The model under review builds one solid part; all positions refer to its coordinate system, in mm. Coordinates: 2 decimals unless noted, no trailing zeros. Order: outer loops, then holes, each group sorted by start corner. A loop starts at its lowest first (then second) coordinate and runs counter-clockwise, first axis right, second up. Notation, with made-up numbers: (74.25, 89.25) - (125.25, 89.25) arc R21 ccw to (125.25, 94.25) - close; hole circle Ø5 at (-26.5, 66). An arc over 180 degrees is marked (long way). Answer in a Markdown table with one row per item.
Autodesk Inventor part; units mm, degrees
ref_plane "YZ Plane" through (0, 0, 0) normal (1, 0, 0) x (0, 1, 0)
ref_plane "XZ Plane" through (0, 0, 0) normal (0, 1, 0) x (-1, 0, 0)
ref_plane "XY Plane" through (0, 0, 0) normal (0, 0, 1) x (1, 0, 0)
sketch "Sketch1" plane through (0, 0, 0) normal (0, 0, 1) x (1, 0, 0)
  line L0 (0, 3.85) -> (0, -3.85)
  line L1 (0, -3.85) -> (4, -3.85)
  line L2 (4, -3.85) -> (4, 3.85)
  line L3 (4, 3.85) -> (0, 3.85)
  arc A0 (0, -5.5518) -> (0, 5.5518) centre (0, 0) ccw
  line L4 (0, 5.5518) -> (0, -5.5518)
  line L5 (4, 5.5518) -> (6, 5.5518)
  line L6 (6, 5.5518) -> (6, -5.5518)
  line L7 (6, -5.5518) -> (4, -5.5518)
  line L8 (4, -5.5518) -> (4, 5.5518)
  line L9 (0, 2.5) -> (6, 2.5)
  line L10 (6, 2.5) -> (6, 0)
  line L11 (6, 0) -> (0, 0)
  line L12 (0, 0) -> (0, 2.5)
  dimension "d0" = 7.7
  dimension "d2" = 4
  dimension "d3" = 3.85
  dimension "d4" = 2
  dimension "d5" = 2
  dimension "d6" = 6
  dimension "d7" = 6
  dimension "d8" = 2.5
  dimension "d9" = 2.5
revolve "Revolution1" add sketch "Sketch1" angle 360 about axis through (0, 5.5518, 0) along (0, -1, 0) contours L3 L2 L9 L0 | L4 A0 L3 | L9 L2 L11 L0 | A0 L9 L2 | L11 L2 L1 L0 | L9 A0 L11 L2 | L1 A0 L4 | L11 A0 L2
extrude "Extrusion1" cut sketch "Sketch1" along normal mid plane 10 contours A0 L9 L2 | L8 L5 L6 L9 A0 | L9 A0 L11 L2 | L9 L6 L11 A0 | L11 A0 L2 | L11 L6 L7 L8 A0
mirror "Mirror1" about plane through (0, 0, 0) normal (1, 0, 0) of "Extrusion1"
revolve "Revolution2" cut sketch "Sketch1" angle 360 about axis through (6, 0, 0) along (-1, 0, 0) contours L9 L2 L11 L0 | L9 A0 L11 L2 | L9 L6 L11 A0
mirror "Mirror2" about plane through (0, 1.25, 0) normal (1, 0, 0) of "Revolution2"
chamfer "Chamfer1" distance 0.5 angle 45 2 edges at (-4, -2.5, 0) (4, -2.5, 0)
properties part number "KULA" material "Stainless Steel"
Item 1: We need section C-C, the plane y = 4. Write out the cut boundary in (x, z).
Check values:
| item | result |
|---|---|
| outline | circle Ø7.7 at (0, 0) |
Item 2: We need section D-D, the plane z = -3.25. Write out the cut boundary in (x, y).
Check values:
| item | result |
|---|---|
| outline | (-4, -2.06) arc R4.5 ccw to (4, -2.06) - (4, 2.06) arc R4.5 ccw to (-4, 2.06) - close |
Item 3: Mouldability with a two-part tool opening along Y and no side actions: class faces 1 (the face through (-0.05, -0.54, 2.44)), 2 (the face through (-4, 1, 3)) as +Y half, -Y half, draft (parallel to the pull), parting line (faces both ways), or undercut.
Check values:
| item | result |
|---|---|
| face 1 | undercut |
| face 2 | draft |
Item 4: We need section A-A, the plane y = 0. Write out the cut boundary in (x, z), then the cut area to 3 significant figures.
Check values:
| item | result |
|---|---|
| outline | (-4, -3.85) arc R5.55 ccw to (4, -3.85) - (4, -3) - (3.5, -2.5) - (-3.5, -2.5) - (-4, -3) - close; (-4, 3) - (-3.5, 2.5) - (3.5, 2.5) - (4, 3) - (4, 3.85) arc R5.55 ccw to (-4, 3.85) - close |
| area | 39.9 mm^2 |
Item 5: We need section B-B, the plane x = 3. Write out the cut boundary in (y, z).
Check values:
| item | result |
|---|---|
| outline | circle Ø9.34 at (0, 0); hole circle Ø5 at (0, 0) |
Item 6: To check wall thickness, follow line 1 (Y direction, x = -2, z = 0); line 2 (Z direction, x = 2.75, y = 1.5); line 3 (Y direction, x = -0.5, z = 2). State the ranges of each line that lie inside material, in increasing order. Write a range as from..to.
Check values:
| item | result |
|---|---|
| line 1 | -5.18..-2.5, 2.5..5.18 |
| line 2 | -4.58..-2, 2..4.58 |
| line 3 | -5.15..-1.5, 1.5..5.15 |
Item 7: Clearance check with flat-ended pins moving along their axes: pin 1 Ø4 at (x, y) = (-0.5, 2) entering from +Z; pin 2 Ø4 at (x, y) = (0, -0.5) entering from -Z; pin 3 Ø2 at (x, y) = (-3, 0) entering from +Z. State where each tip first meets the part, or that it passes through.
Check values:
| item | result |
|---|---|
| pin 1 | z = 5.55 |
| pin 2 | z = -5.55 |
| pin 3 | z = 5.18 |
